Input: part model. Units: mm. Frame: model coordinates. A direction names the side the tool comes from. Coordinates: 2 decimals unless noted, no trailing zeros. Order: outer loops, then holes, each group sorted by start corner. A loop starts at its lowest first (then second) coordinate and runs counter-clockwise, first axis right, second up.
from build123d import *

# Parameters (mm, degrees)
SKETCH_1_R      = 14
EXTRUDE_1_DEPTH = 19
SKETCH_2_R      = 2.1
EXTRUDE_2_DEPTH = 1
SKETCH_3_R      = 4.5
EXTRUDE_3_DEPTH = 1.5
SKETCH_4_R      = 2.5
EXTRUDE_4_DEPTH = 2.5
EXTRUDE_5_DEPTH = 6


with BuildPart() as part:
    # 草图1 → 凸台-拉伸1 (new body)
    with BuildSketch(Plane(origin=(0, 0, 0), x_dir=(1, 0, 0), z_dir=(0, 1, 0))):
        with Locations(Location((0, 0, 0), (0, 0, 270))):
            Circle(SKETCH_1_R)
    extrude(amount=EXTRUDE_1_DEPTH)

    # 草图2 → 凸台-拉伸2 (add)
    with BuildSketch(Plane(origin=(0, 19, 0), x_dir=(1, 0, 0), z_dir=(0, 1, 0))):
        with BuildLine():
            Line((-17.5, 3.5), (17.5, 3.5))
            ThreePointArc((17.5, 3.5), (21, 0), (17.5, -3.5))
            Line((17.5, -3.5), (-17.5, -3.5))
            ThreePointArc((-17.5, -3.5), (-21, 0), (-17.5, 3.5))
        make_face()
        with Locations(Location((-17.5, 0, 0), (0, 0, 270))):
            Circle(SKETCH_2_R, mode=Mode.SUBTRACT)
        with Locations(Location((17.5, 0, 0), (0, 0, 270))):
            Circle(SKETCH_2_R, mode=Mode.SUBTRACT)
    extrude(amount=-EXTRUDE_2_DEPTH)

    # 草图3 → 凸台-拉伸3 (add)
    with BuildSketch(Plane(origin=(0, 19, 0), x_dir=(1, 0, 0), z_dir=(0, 1, 0))):
        with Locations(Location((0, 8, 0), (0, 0, 270))):
            Circle(SKETCH_3_R)
    extrude(amount=EXTRUDE_3_DEPTH)

    # 草图4 → 凸台-拉伸4 (add)
    with BuildSketch(Plane(origin=(0, 20.5, 0), x_dir=(1, 0, 0), z_dir=(0, 1, 0))):
        with Locations(Location((0, 8, 0), (0, 0, 270))):
            Circle(SKETCH_4_R)
    extrude(amount=EXTRUDE_4_DEPTH)

    # 草图5 → 凸台-拉伸5 (add)
    with BuildSketch(Plane(origin=(0, 23, 0), x_dir=(1, 0, 0), z_dir=(0, 1, 0))):
        with BuildLine():
            Line((-1.5, 10), (-1.5, 6))
            ThreePointArc((-1.5, 6), (0, 5.5), (1.5, 6))
            Line((1.5, 6), (1.5, 10))
            ThreePointArc((1.5, 10), (0, 10.5), (-1.5, 10))
        make_face()
    extrude(amount=EXTRUDE_5_DEPTH)


solid = part.part
Item 1: Cut plane D-D on y = 7. Return loops of the section in (x, z), then the cut area to 3 significant figures.
Response values:
outline: circle Ø28 at (0, 0)
area: 616 mm2
Item 2: Draft query along Z for faces 1 (the face through (0, 0, 0)), 2 (the face through (15.6, 18.5, 3.5)), 3 (the face through (-15.418, 18.507, -0.273)). Return one class per face: pulls with the +Z half, pulls with the -Z half, needs draft (parallel to the pull), parting line crosses it, or undercut.
Response values:
face 1: needs draft
face 2: pulls with the +Z half
face 3: undercut
Item 3: Ray query, probe 1 along X at (y, z) = (18.4, 0); probe 2 along Y at (x, z) = (10.5, -3); probe 3 along Y at (x, z) = (14.5, 2). Return the intervals inside material, ascending.
Response values:
probe 1: x = -21 to -19.6, -15.4 to 15.4, 19.6 to 21
probe 2: y = 0 to 19
probe 3: y = 18 to 19
Item 4: Pin query (flat end, axial travel): pin 1 Ø0.8 at (x, z) = (2, -7.5) entering from +Y; pin 2 Ø3.5 at (x, z) = (-16.5, -0.5) entering from -Y; pin 3 Ø4 at (x, z) = (-7.5, 1.5) entering from +Y; pin 4 Ø2.5 at (x, z) = (-17.5, 0) entering from +Y. Return the tip coordinate at first contact, or that it passes through.
Response values:
pin 1: stops at y = 23
pin 2: stops at y = 18
pin 3: stops at y = 19
pin 4: passes through
Item 5: Cut plane C-C on z = -7.5. Return loops of the section in (x, y).
Response values:
outline: (-11.82, 0) - (11.82, 0) - (11.82, 19) - (4.47, 19) - (4.47, 20.5) - (2.45, 20.5) - (2.45, 23) - (1.5, 23) - (1.5, 29) - (-1.5, 29) - (-1.5, 23) - (-2.45, 23) - (-2.45, 20.5) - (-4.47, 20.5) - (-4.47, 19) - (-11.82, 19) - close
Item 6: Access query for faces 4 (the face through (-15.5, 18.5, 3.5)), 5 (the face through (-15.6, 18.5, -3.5)), 6 (the face through (1.5, 26, -8)), 7 (the face through (1.352, 19.74, -3.708)). Directions: +Z, -Z, +X, -X, +Y, -Y. A direction counts if a zero-diameter tool reaches every point of the face in a straight line with its end or side. Return the directions, or none.
Response values:
face 4: +Z, -X, +Y, -Y
face 5: -Z, -X, +Y, -Y
face 6: +Z, -Z, +X, +Y
face 7: +Y
Item 7: Cut plane A-A on z = 0. Return loops of the section in (x, y), then the cut area to 3 significant figures.
Response values:
outline: (-21, 18) - (-19.6, 18) - (-19.6, 19) - (-21, 19) - close; (-15.4, 18) - (-14, 18) - (-14, 0) - (14, 0) - (14, 18) - (15.4, 18) - (15.4, 19) - (-15.4, 19) - close; (19.6, 18) - (21, 18) - (21, 19) - (19.6, 19) - close
area: 538 mm2
Item 8: Cut plane B-B on x = -16.5. Return loops of the section in (y, z), then the cut area to 3 significant figures.
Response values:
outline: (18, -3.5) - (19, -3.5) - (19, -1.85) - (18, -1.85) - close; (18, 1.85) - (19, 1.85) - (19, 3.5) - (18, 3.5) - close
area: 3.31 mm2
